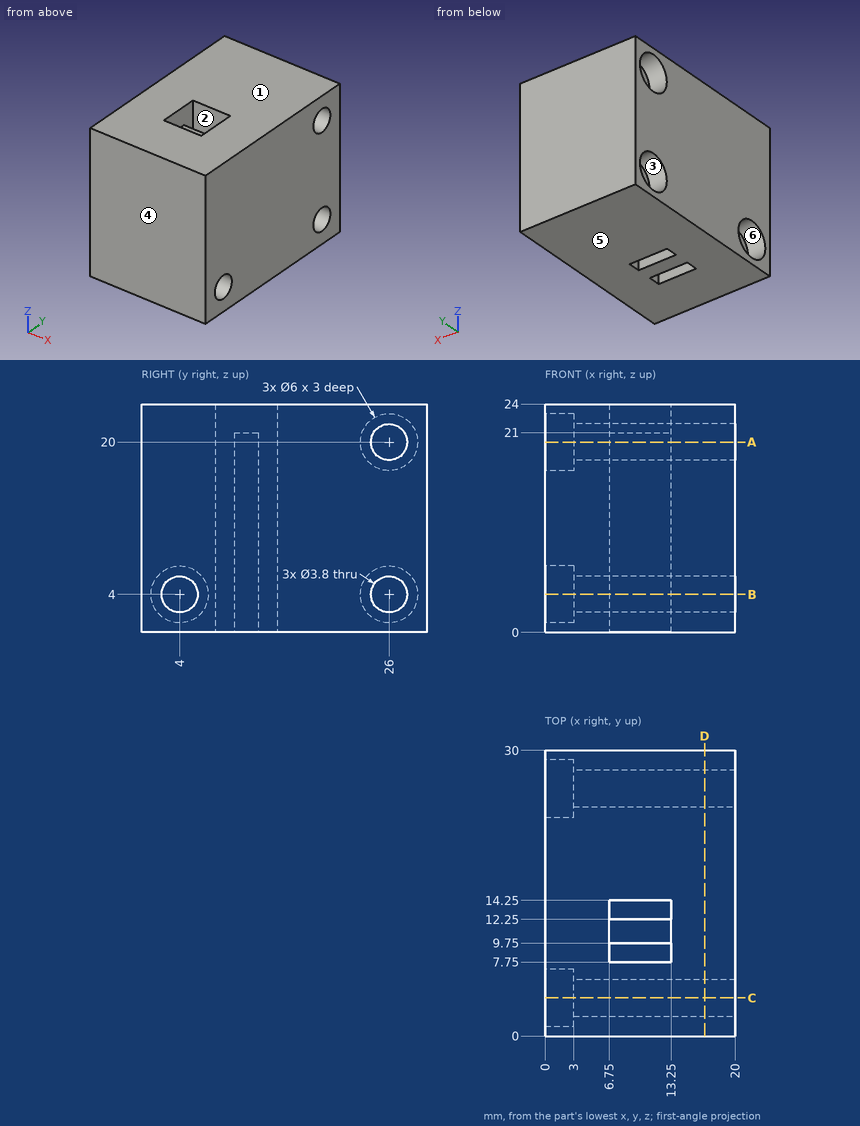
Job drawing, mm, ordinate dimensions from the low corner. One solid piece. A direction names the side the tool comes from. Coordinates: 2 decimals unless noted, no trailing zeros. Order: outer loops, then holes, each group sorted by start corner. A loop starts at its lowest first (then second) coordinate and runs counter-clockwise, first axis right, second up. Notation, with made-up numbers: (-33.75, 37) -> (-17.75, 37) arc R18 cw to (-17.75, 67) -> close; hole circle Ø10 at (25, -26). An arc over 180 degrees is marked (long way). Put each result on its own line as item: value. Start each with the question number.
(1) Probe line 1 along Z through (x, y) = (7.75, 26); line 2 along Z through (x, y) = (1.4, 26); line 3 along Y through (x, z) = (11.25, 16.5). List the from-to ranges inside material, lowest first. Write a range as [from, to].
(2) Band-saw the part on A-A (z = 20). Give the cut face in (x, y), then the cut area to 3 significant figures.
(3) Which spindle directions (+Z, -Z, +X, -X, +Y, -Y) get a long thin tool onto all of the face, cutting with end or side? Do the marked faces 1, 2 and 3. Say none if no direction does.
(4) Band-saw the part on D-D (x = 16.75). Give the cut face in (y, z).
(5) Pin check, flat tip, straight feed: pin 1 Ø1.8 at (y, z) = (25.5, 19) entering from -X. Stop position of the tip, or through.
(6) Mould opens along Z. For the marked faces 4, 5 and 6 say: pulls with the +Z half, pulls with the -Z half, needs draft (parallel to the pull), parting line crosses it, or undercut.
(7) Band-saw the part on B-B (z = 4). Give the cut face in (x, y).
(8) Band-saw the part on C-C (y = 4). Give the cut face in (x, z), then the cut area to 3 significant figures.
Determined:
1. line 1: z = [0, 2.1], [5.9, 18.1], [21.9, 24]
1. line 2: z = [0, 1], [7, 17], [23, 24]
1. line 3: y = [0, 7.75], [9.75, 12.25], [14.25, 30]
2. outline: (0, 0) -> (20, 0) -> (20, 24.1) -> (3, 24.1) -> (3, 23) -> (0, 23) -> close; (0, 29) -> (3, 29) -> (3, 27.9) -> (20, 27.9) -> (20, 30) -> (0, 30) -> close; hole (6.75, 7.75) -> (13.25, 7.75) -> (13.25, 9.75) -> (6.75, 9.75) -> close; hole (6.75, 12.25) -> (13.25, 12.25) -> (13.25, 14.25) -> (6.75, 14.25) -> close
2. area: 491 mm²
3. face 1: +Z, +X, -X, +Y, -Y
3. face 2: +Z, -Z
3. face 3: -X
4. outline: (0, 0) -> (30, 0) -> (30, 24) -> (0, 24) -> close; hole circle Ø3.8 at (4, 4); hole circle Ø3.8 at (26, 4); hole circle Ø3.8 at (26, 20)
5. pin 1: stops at x = 3
6. face 4: needs draft
6. face 5: pulls with the -Z half
6. face 6: undercut
7. outline: (0, 0) -> (20, 0) -> (20, 2.1) -> (3, 2.1) -> (3, 1) -> (0, 1) -> close; (0, 7) -> (3, 7) -> (3, 5.9) -> (20, 5.9) -> (20, 24.1) -> (3, 24.1) -> (3, 23) -> (0, 23) -> close; (0, 29) -> (3, 29) -> (3, 27.9) -> (20, 27.9) -> (20, 30) -> (0, 30) -> close; hole (6.75, 7.75) -> (13.25, 7.75) -> (13.25, 9.75) -> (6.75, 9.75) -> close; hole (6.75, 12.25) -> (13.25, 12.25) -> (13.25, 14.25) -> (6.75, 14.25) -> close
8. outline: (0, 0) -> (20, 0) -> (20, 2.1) -> (3, 2.1) -> (3, 1) -> (0, 1) -> close; (0, 7) -> (3, 7) -> (3, 5.9) -> (20, 5.9) -> (20, 24) -> (0, 24) -> close
8. area: 397 mm²
